Can you work these out from the model? Positions are in its coordinate system, mm. Face numbers are marked on the shaded views. A direction names the side the tool comes from. Give positions to 0.01 mm unless a question says otherwise; leave off trailing zeros. Order: outer loops, then holes, each group sorted by start corner. A loop starts at its lowest first (then second) coordinate and runs counter-clockwise, first axis right, second up.
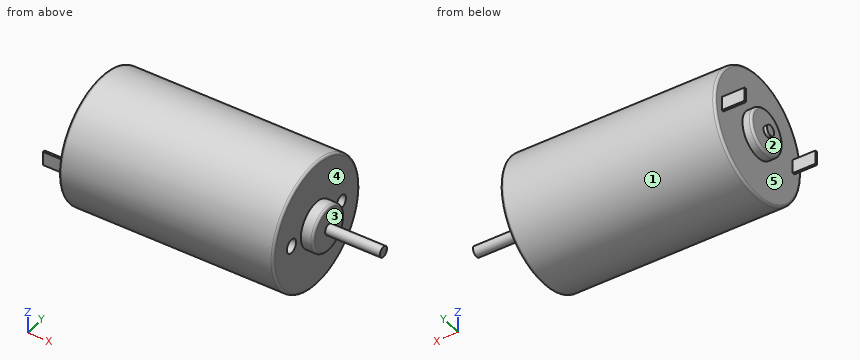
```python
from build123d import *

# Parameters (mm, degrees)
SKETCH1_R           = 13.85
BOSS_EXTRUDE1_DEPTH = 47
SKETCH2_R           = 5
BOSS_EXTRUDE2_DEPTH = 2.7
SKETCH3_R           = 1.15
BOSS_EXTRUDE3_DEPTH = 12
SKETCH4_R           = 5
BOSS_EXTRUDE4_DEPTH = 2
SKETCH5_R           = 1.15
BOSS_EXTRUDE5_DEPTH = 0.75
SKETCH6_W           = 3
SKETCH6_H           = 0.5
BOSS_EXTRUDE6_DEPTH = 5
SKETCH7_R           = 1.5
CUT_EXTRUDE1_DEPTH  = 5
FILLET1_R           = 0.5


with BuildPart() as part:
    # Sketch1 → Boss-Extrude1 (new body)
    with BuildSketch(Plane(origin=(0, 0, 0), x_dir=(0, 0, -1), z_dir=(1, 0, 0))):
        Circle(SKETCH1_R)
    extrude(amount=BOSS_EXTRUDE1_DEPTH)

    # Sketch2 → Boss-Extrude2 (add)
    with BuildSketch(Plane(origin=(47, 0, 0), x_dir=(0, 0, -1), z_dir=(1, 0, 0))):
        Circle(SKETCH2_R)
    extrude(amount=BOSS_EXTRUDE2_DEPTH)

    # Sketch3 → Boss-Extrude3 (add)
    with BuildSketch(Plane(origin=(49.7, 0, 0), x_dir=(0, 0, -1), z_dir=(1, 0, 0))):
        Circle(SKETCH3_R)
    extrude(amount=BOSS_EXTRUDE3_DEPTH)

    # Sketch4 → Boss-Extrude4 (add)
    with BuildSketch(Plane.ZY):
        Circle(SKETCH4_R)
    extrude(amount=BOSS_EXTRUDE4_DEPTH)

    # Sketch5 → Boss-Extrude5 (add)
    with BuildSketch(Plane.ZY.offset(2)):
        Circle(SKETCH5_R)
    extrude(amount=BOSS_EXTRUDE5_DEPTH)

    # Sketch6 → Boss-Extrude6 (add)
    with BuildSketch(Plane.ZY):
        with Locations((0, 11.4)):
            Rectangle(SKETCH6_W, SKETCH6_H)
        with Locations((0, -11.4)):
            Rectangle(SKETCH6_W, SKETCH6_H)
    extrude(amount=BOSS_EXTRUDE6_DEPTH)

    # Sketch7 → Cut-Extrude1 (cut)
    with BuildSketch(Plane(origin=(47, 0, 0), x_dir=(0, 0, -1), z_dir=(1, 0, 0))):
        with Locations((0, 8)):
            Circle(SKETCH7_R)
        with Locations((0, -8)):
            Circle(SKETCH7_R)
    extrude(amount=-CUT_EXTRUDE1_DEPTH, mode=Mode.SUBTRACT)

    # Fillet1
    fillet1_edges = [part.edges().sort_by_distance(p)[0] for p in [
        (-2, 0, -5),
        (0, 0, 13.85),
        (47, 0, 13.85),
        (49.7, 0, 5),
    ]]
    fillet(fillet1_edges, radius=FILLET1_R)


solid = part.part
```
1) If I drill on line 1 (Y direction, x = 45.6, z = 0); line 2 (X direction, y = -9.5, z = 4); line 3 (X direction, y = -3.75, z = -1.5), over which ranges is the centre line in solid material (lowest first)?
2) I'm going to push flat-ended pins straight in: pin 1 Ø1.5 at (x, z) = (-3, 0.5) entering from +Y; pin 2 Ø2.5 at (x, z) = (-1.5, -0.5) entering from -Y; pin 3 Ø1 at (y, z) = (-3.5, -3) entering from -X. Where does each tip first touch, or does it pass through?
3) Suppose I cut it at B-B (x = 23.5). Please give me the cut outline in (y, z).
4) We'd pull the mould along Y, two halves only. Please class the marked faces 1, 2 and 3: +Y half, -Y half, draft (parallel to the pull), parting line (faces both ways), or undercut.
5) Suppose I cut it at A-A (y = 0). Please give me the cut outline in (x, z), and give its area (3 significant figures).
6) Which directions (+Z, -Z, +X, -X, +Y, -Y) give clear straight access to the entire face, cutting with the end or side of a thin tool? Please do the marked faces 4 and 5.
Results:
1. line 1: y = -13.85 to -9.5, -6.5 to 6.5, 9.5 to 13.85
1. line 2: x = 0 to 47
1. line 3: x = -2 to 49.7
2. pin 1: stops at y = 11.65
2. pin 2: stops at y = -11.65
2. pin 3: stops at x = -2
3. outline: circle Ø27.7 at (0, 0)
4. face 1: parting line
4. face 2: undercut
4. face 3: draft
5. outline: (-2.75, -1.15) - (-2, -1.15) - (-2, -4.5) arc R0.5 ccw to (-1.5, -5) - (0, -5) - (0, -13.35) arc R0.5 ccw to (0.5, -13.85) - (46.5, -13.85) arc R0.5 ccw to (47, -13.35) - (47, -5) - (49.2, -5) arc R0.5 ccw to (49.7, -4.5) - (49.7, -1.15) - (61.7, -1.15) - (61.7, 1.15) - (49.7, 1.15) - (49.7, 4.5) arc R0.5 ccw to (49.2, 5) - (47, 5) - (47, 13.35) arc R0.5 ccw to (46.5, 13.85) - (0.5, 13.85) arc R0.5 ccw to (0, 13.35) - (0, 5) - (-1.5, 5) arc R0.5 ccw to (-2, 4.5) - (-2, 1.15) - (-2.75, 1.15) - close
5. area: 1,380 mm2
6. face 4: +X
6. face 5: -X
